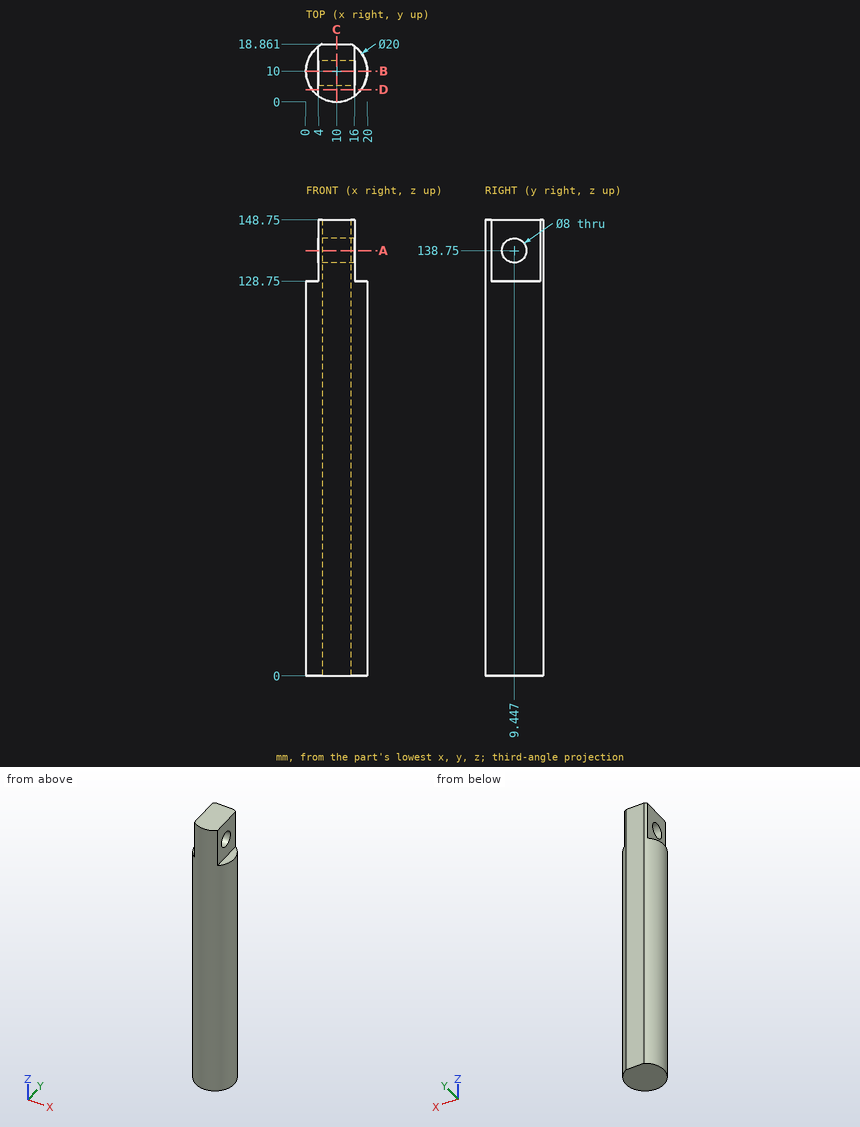
Check sheet for the drawn part. Datum: minimum x, y, z corner. Units: mm. Coordinates: 2 decimals unless noted, no trailing zeros. Loops run counter-clockwise (first coordinate to the right, second up) from the corner with the lowest first, then second, coordinate; pieces in that order, holes last. Notation, with made-up numbers: M 52,87.5 L 73,87.5 A15 cw 73,99.5 Z; hole C 44,33 d6. An arc over 180 degrees is marked long. Answer as a JSON object with one key per item and string values.
1. Sectioned sample at C-C on x = 10. Record the cut outline in (y, z), and give its area (3 significant figures).
Outcome:
{"outline": "M 0,0 L 18.86,0 L 18.86,148.75 L 0,148.75 Z; hole C 9.45,138.75 d8", "area": "2,760 mm²"}
2. Depth check by flat-ended pin: P1, Ø1, axis at y = 15.5, z = 107.5, coming from the -X side; P2, Ø3, axis at x = 13.5, z = 90, coming from the -Y side; P3, Ø2, axis at y = 7, z = 108, coming from the +X side; P4, Ø6.5, axis at y = 9.45, z = 138.75, coming from the -X side. Enter the tip coordinate at first touch or a pass-through.
Outcome:
{"P1": "x = 1.34", "P2": "y = 0.2", "P3": "x = 19.8", "P4": "through"}
3. Sectioned sample at D-D on y = 4. Record the cut outline in (x, z).
Outcome:
{"outline": "M 2,0 L 18,0 L 18,128.75 L 16,128.75 L 16,148.75 L 4,148.75 L 4,128.75 L 2,128.75 Z"}
4. Sectioned sample at A-A on z = 138.75. Record the cut outline in (x, y) (1 decimal).
Outcome:
{"outline": "M 4,2 A10 ccw 16,2 L 16,5.4 L 4,5.4 Z; M 4,13.4 L 16,13.4 L 16,18 A10 ccw 14.6,18.9 L 5.4,18.9 A10 ccw 4,18 Z"}
5. Sectioned sample at B-B on y = 10. Record the cut outline in (x, z), and give its area (3 significant figures).
Outcome:
{"outline": "M 0,0 L 20,0 L 20,128.75 L 16,128.75 L 16,134.79 L 4,134.79 L 4,128.75 L 0,128.75 Z; M 4,142.71 L 16,142.71 L 16,148.75 L 4,148.75 Z", "area": "2,720 mm²"}
6. Scan lines: L1, parallel to Y at x = 9.5, z = 132; L2, parallel to X at y = 10.5, z = 90; L3, parallel to Z at x = 16.75, y = 5. Record each from-to range of solid material in increasing order. Write a range as from..to.
Outcome:
{"L1": "0.01..18.86", "L2": "0.01..19.99", "L3": "0..128.75"}
